Model file for the job. Use its own axes, mm. A direction names the side the tool comes from. Round coordinates to 2 decimals unless told otherwise and drop trailing zeros. Order: outer loops, then holes, each group sorted by start corner. A loop starts at its lowest first (then second) coordinate and runs counter-clockwise, first axis right, second up. Notation, with made-up numbers: (18.5, -18) - (64.5, -18) arc R12 cw to (64.5, -13) - close; hole circle Ø4 at (-28, 57.5). An arc over 180 degrees is marked (long way). Put each result on its own line as item: value. Start each with the question number.
Item 1: Probe probe 1 along X at (y, z) = (18, 54); probe 2 along Z at (x, y) = (7, 36); probe 3 along Y at (x, z) = (8, 87). List the from-to ranges inside material, lowest first.
Item 2: Saw through at A-A on x = 26. List the corners of the cut face in (y, z), plus the area to 3 significant figures.
Item 3: Which spindle directions (+Z, -Z, +X, -X, +Y, -Y) get a long thin tool onto all of the face, cutting with end or side? Do faces 5 (the face through (35.43, 59.23, 49.3)), 6 (the face through (12.564, 53.517, 49.3)). Say none if no direction does.
Item 4: Mould opens along Z. For faces 1 (the face through (5.42, 28.96, 90.09)), 2 (the face through (46.42, 28.96, 90.09)), 3 (the face through (17, 55, 49)), 4 (the face through (8, 24, 100)) say: pulls with the +Z half, pulls with the -Z half, needs draft (parallel to the pull), parting line crosses it, or undercut.
Item 5: Saw through at B-B on y = 22.5. List the corners of the cut face in (x, z).
Item 6: Saw through at C-C on z = 87.5. List the corners of the cut face in (x, y), plus the area to 3 significant figures.
Item 7: Saw through at D-D on y = 33.5. List the corners of the cut face in (x, z).
Item 8: Pin check, flat tips, straight feed: pin 1 Ø6 at (x, z) = (22, 14.5) entering from +Y; pin 2 Ø10 at (y, z) = (44, 10.5) entering from +X; pin 3 Ø9 at (y, z) = (36, 87.5) entering from -X; pin 4 Ø2 at (y, z) = (52.5, 47.5) entering from +X. Stop position of each tip, or through.
```python
from build123d import *

# Parameters (mm, degrees)
BOSS_EXTRUDE1_DEPTH     = 100
FILLET3_R               = 10
SKETCH2_R               = 7.5
CUT_EXTRUDE1_DEPTH      = 133.680066325
CUT_EXTRUDE5_DEPTH      = 129.160056346
CUT_EXTRUDE5_DEPTH_BACK = 129.160056346
SKETCH3_R               = 7.5


with BuildPart() as part:
    # Sketch1 → Boss-Extrude1 (new body)
    with BuildSketch(Plane.XY):
        with BuildLine():
            Line((0, 35), (0, 0))
            Line((0, 0), (52, 0))
            Line((52, 0), (52, 35))
            ThreePointArc((52, 35), (26, 61), (0, 35))
        make_face()
        with BuildLine():
            Line((11, 49.8), (11, 10.2))
            ThreePointArc((11, 10.2), (12.523044738, 6.523044738), (16.2, 5))
            Line((16.2, 5), (35.8, 5))
            ThreePointArc((35.8, 5), (39.476955262, 6.523044738), (41, 10.2))
            Line((41, 10.2), (41, 49.8))
            ThreePointArc((41, 49.8), (39.476955262, 53.476955262), (35.8, 55))
            Line((35.8, 55), (16.2, 55))
            ThreePointArc((16.2, 55), (12.523044738, 53.476955262), (11, 49.8))
        make_face(mode=Mode.SUBTRACT)
    extrude(amount=BOSS_EXTRUDE1_DEPTH)

    # Fillet3
    fillet3_edges = [part.edges().sort_by_distance(p)[0] for p in [
        (52, 0, 50),
        (0, 0, 50),
    ]]
    fillet(fillet3_edges, radius=FILLET3_R)

    # Sketch2 → Cut-Extrude1 (cut, through all)
    with BuildSketch(Plane(origin=(0, 70, 0), x_dir=(1, 0, 0), z_dir=(0, 1, 0))):
        with Locations(Location((26, -50, 0), (0, 0, 270))):
            Circle(SKETCH2_R)
    extrude(amount=-CUT_EXTRUDE1_DEPTH, mode=Mode.SUBTRACT)

    # Sketch3 → Cut-Extrude5 (cut, two sides: drawn at the far end of the back side and taken through both)
    with BuildSketch(Plane(origin=(0, 0, 0), x_dir=(0, 0, -1), z_dir=(1, 0, 0)).offset(-CUT_EXTRUDE5_DEPTH_BACK)):
        with Locations(Location((-87.5, 36, 0), (0, 0, 352.337744339))):
            Circle(SKETCH3_R)
    extrude(amount=CUT_EXTRUDE5_DEPTH + CUT_EXTRUDE5_DEPTH_BACK, mode=Mode.SUBTRACT)


solid = part.part
```
Results found:
1. probe 1: x = 0 to 11, 41 to 52
1. probe 2: z = 0 to 80, 95 to 100
1. probe 3: y = 0.2 to 28.52, 43.48 to 53.76
2. outline: (0, 0) - (5, 0) - (5, 42.5) - (0, 42.5) - close; (0, 57.5) - (5, 57.5) - (5, 100) - (0, 100) - close; (55, 0) - (61, 0) - (61, 42.5) - (55, 42.5) - close; (55, 57.5) - (61, 57.5) - (61, 100) - (55, 100) - close
2. area: 935 mm²
3. face 5: +Z, -Z, +Y
3. face 6: +Z, -Z
4. face 1: undercut
4. face 2: undercut
4. face 3: needs draft
4. face 4: pulls with the +Z half
5. outline: (0, 0) - (11, 0) - (11, 100) - (0, 100) - close; (41, 0) - (52, 0) - (52, 100) - (41, 100) - close
6. outline: (0, 10) arc R10 ccw to (10, 0) - (42, 0) arc R10 ccw to (52, 10) - (52, 28.5) - (41, 28.5) - (41, 10.2) arc R5.2 cw to (35.8, 5) - (16.2, 5) arc R5.2 cw to (11, 10.2) - (11, 28.5) - (0, 28.5) - close; (1.43, 43.5) - (11, 43.5) - (11, 49.8) arc R5.2 cw to (16.2, 55) - (35.8, 55) arc R5.2 cw to (41, 49.8) - (41, 43.5) - (50.57, 43.5) arc R26 ccw to start
6. area: 1,040 mm²
7. outline: (0, 0) - (11, 0) - (11, 80.43) - (0, 80.43) - close; (0, 94.57) - (11, 94.57) - (11, 100) - (0, 100) - close; (41, 0) - (52, 0) - (52, 80.43) - (41, 80.43) - close; (41, 94.57) - (52, 94.57) - (52, 100) - (41, 100) - close
8. pin 1: stops at y = 60.98
8. pin 2: stops at x = 51.69
8. pin 3: passes through
8. pin 4: stops at x = 46.09
